For this review, take the finished solid that the model builds, in its own axes (mm). Face numbers are marked on the shaded views. A direction names the side the tool comes from. Give positions to 0.01 mm unless a question says otherwise; leave off trailing zeros. Order: outer loops, then holes, each group sorted by start corner. A loop starts at its lowest first (then second) coordinate and runs counter-clockwise, first axis right, second up. Notation, with made-up numbers: M 73,62.5 L 120,62.5 A9 cw 120,66.5 Z; hole C 13.5,73 d9. An arc over 180 degrees is marked long. Answer as CSV lines item,"result". Start each with the question number.
1. Machinability: for the marked faces 4, 5, 6 and 7, which of the approach directions +Z, -Z, +X, -X, +Y, -Y give a long, thin tool a straight path to every point of the face, cutting with its end or side? Answer none if there is none.
2. We need section B-B, the plane y = 5. Give the boundary of the cut face in (x, z) (3 decimals), and give its area (3 significant figures).
3. We need section C-C, the plane x = -8.5. Give the boundary of the cut face in (y, z) (3 decimals), and give its area (3 significant figures).
4. We need section D-D, the plane x = -17. Give the boundary of the cut face in (y, z) (1 decimal).
5. We need section A-A, the plane z = -1.5. Give the boundary of the cut face in (x, y) (3 decimals), and give its area (3 significant figures).
6. Clearance check with flat-ended pins moving along their axes: P1, Ø4, axis at y = 23.5, z = 5, coming from the -X side (3 decimals); P2, Ø1, axis at y = 21.5, z = -4, coming from the -X side; P3, Ø16, axis at x = -18.5, z = 2.5, coming from the +Y side (3 decimals). State where each tip first meets the part, or that it passes through.
7. For line 1 along Z through (x, y) = (-25.5, 5); line 2 along X through (y, z) = (5, -2.5) (3 decimals); line 3 along Z through (x, y) = (-10, 33.5), list the stretches that pass through material, from the lowest coordinate up.
8. Mouldability with a two-part tool opening along Y and no side actions: class the marked faces 1, 2 and 3 as pulls with the +Y half, pulls with the -Y half, needs draft (parallel to the pull), parting line crosses it, or undercut.
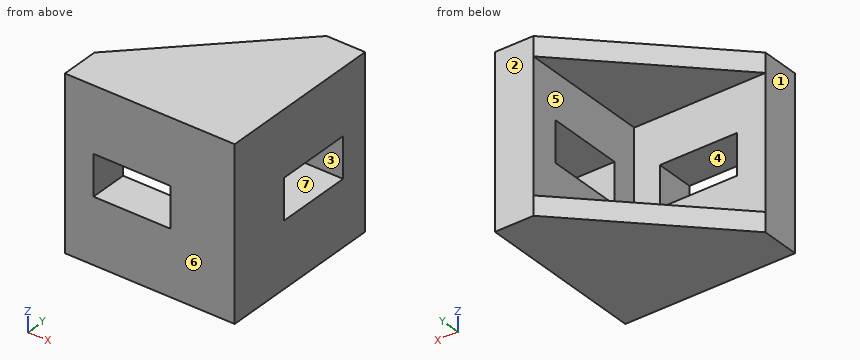
from build123d import *

# Parameters (mm, degrees)
BOSS_EXTRUDE1_DEPTH = 21
BOSS_EXTRUDE2_DEPTH = 4.7625
SKETCH3_W           = 19.05
SKETCH3_H           = 10
CUT_EXTRUDE1_DEPTH  = 10.525


with BuildPart() as part:
    # Sketch1 → Boss-Extrude1 (new body)
    with BuildSketch(Plane.XY):
        Polygon((0, 0), (-42, 0), (-42, 9.525), (-9.525, 9.525), (-9.525, 42), (0, 42), align=None)
    boss_extrude1 = extrude(amount=BOSS_EXTRUDE1_DEPTH)

    # Sketch2 → Boss-Extrude2 (add)
    with BuildSketch(Plane.XY.offset(21)):
        Polygon((-9.525, 42), (-42, 9.525), (-9.525, 9.525), align=None)
    boss_extrude2 = extrude(amount=-BOSS_EXTRUDE2_DEPTH)

    # Mirror1: Boss-Extrude1, Boss-Extrude2 across plane
    add(boss_extrude1.mirror(Plane(origin=(0, 0, 0), x_dir=(1, 0, 0), z_dir=(0, 0, -1))))
    add(boss_extrude2.mirror(Plane(origin=(0, 0, 0), x_dir=(1, 0, 0), z_dir=(0, 0, -1))))

    # Sketch3 → Cut-Extrude1 (cut, through all)
    with BuildSketch(Plane(origin=(0, 9.525, 0), x_dir=(1, 0, 0), z_dir=(0, 1, 0))):
        with Locations((-25.4, 0)):
            Rectangle(SKETCH3_W, SKETCH3_H)
    cut_extrude1 = extrude(amount=-CUT_EXTRUDE1_DEPTH, mode=Mode.SUBTRACT)

    # Mirror2: Cut-Extrude1 across plane
    add(cut_extrude1.mirror(Plane(origin=(0, 0, 0), x_dir=(0, 0, 1), z_dir=(0.707106781, 0.707106781, 0))), mode=Mode.SUBTRACT)


solid = part.part
Result set:
1,face 4,"+Y, -Y"
1,face 5,"-X, +Y"
1,face 6,"+Z, -Z, +X, -X, -Y"
1,face 7,"+X, -X"
2,outline,"M -42,-21 L 0,-21 L 0,21 L -42,21 Z; hole M -34.925,-5 L -15.875,-5 L -15.875,5 L -34.925,5 Z"
2,area,"1,570 mm2"
3,outline,"M 0,-21 L 42,-21 L 42,21 L 0,21 Z; hole M 15.875,-5 L 34.925,-5 L 34.925,5 L 15.875,5 Z"
3,area,"1,570 mm2"
4,outline,"M 0,-21 L 34.5,-21 L 34.5,-16.2 L 9.5,-16.2 L 9.5,-5 L 0,-5 Z; M 0,5 L 9.5,5 L 9.5,16.2 L 34.5,16.2 L 34.5,21 L 0,21 Z"
5,outline,"M -42,0 L -34.925,0 L -34.925,9.525 L -42,9.525 Z; M -15.875,0 L 0,0 L 0,15.875 L -9.525,15.875 L -9.525,9.525 L -15.875,9.525 Z; M -9.525,34.925 L 0,34.925 L 0,42 L -9.525,42 Z"
5,area,"346 mm2"
6,P1,"x = -9.525"
6,P2,"through"
6,P3,"y = 9.525"
7,line 1,"-21 to -5, 5 to 21"
7,line 2,"-42 to -34.925, -15.875 to 0"
7,line 3,"-21 to -16.24, 16.24 to 21"
8,face 1,"needs draft"
8,face 2,"pulls with the +Y half"
8,face 3,"undercut"
